Autodesk Inventor part; units mm, degrees
ref_plane "YZ Plane" through (0, 0, 0) normal (1, 0, 0) x (0, 1, 0)
ref_plane "XZ Plane" through (0, 0, 0) normal (0, 1, 0) x (-1, 0, 0)
ref_plane "XY Plane" through (0, 0, 0) normal (0, 0, 1) x (1, 0, 0)
sketch "Boceto1" plane through (0, 0, 0) normal (0, 0, 1) x (1, 0, 0)
  circle A0 centre (0, 0) radius 2.1
  line L0 (-12, 0) -> (12, 0)
  line L1 (0, 12) -> (0, -12)
  line L2 (0, 3.9) -> (-2.845, 3.9)
  line L3 (-2.845, 3.9) -> (-5.5, 6.555)
  line L4 (-5.5, 6.555) -> (-5.5, 8.195)
  line L5 (-5.5, 8.195) -> (-3.125, 8.195)
  line L6 (-3.125, 8.545) -> (-4.58, 10)
  line L7 (-4.58, 10) -> (-10, 10)
  line L8 (-10, 10) -> (-10, 4.58)
  line L9 (-10, 4.58) -> (-8.545, 3.125)
  line L10 (-8.195, 3.125) -> (-8.195, 5.4887)
  line L11 (-8.195, 5.4887) -> (-6.555, 5.4887)
  line L12 (-6.555, 5.4887) -> (-3.9, 2.8337)
  line L13 (-3.9, 2.8337) -> (-3.9, 0)
  line L14 (0, 3.9) -> (2.845, 3.9)
  line L15 (2.845, 3.9) -> (5.5, 6.555)
  line L16 (5.5, 6.555) -> (5.5, 8.195)
  line L17 (5.5, 8.195) -> (3.125, 8.195)
  line L18 (3.125, 8.545) -> (4.58, 10)
  line L19 (4.58, 10) -> (10, 10)
  line L20 (10, 10) -> (10, 4.58)
  line L21 (10, 4.58) -> (8.545, 3.125)
  line L22 (8.2079, 3.125) -> (8.195, 5.4887)
  line L23 (8.195, 5.4887) -> (6.555, 5.4887)
  line L24 (6.555, 5.4887) -> (3.9, 2.8337)
  line L25 (3.9, 2.8337) -> (3.9, 0)
  line L26 (0, -3.9) -> (-2.845, -3.9)
  line L27 (-2.845, -3.9) -> (-5.5, -6.555)
  line L28 (-5.5, -6.555) -> (-5.5, -8.195)
  line L29 (-5.5, -8.195) -> (-3.125, -8.195)
  line L30 (-3.125, -8.545) -> (-4.58, -10)
  line L31 (-4.58, -10) -> (-10, -10)
  line L32 (-10, -10) -> (-10, -4.58)
  line L33 (-10, -4.58) -> (-8.545, -3.125)
  line L34 (-8.195, -3.125) -> (-8.195, -5.4887)
  line L35 (-8.195, -5.4887) -> (-6.555, -5.4887)
  line L36 (-6.555, -5.4887) -> (-3.9, -2.8337)
  line L37 (-3.9, -2.8337) -> (-3.9, 0)
  line L38 (10, -10) -> (10, -4.58)
  line L39 (4.58, -10) -> (10, -10)
  line L40 (3.125, -8.545) -> (4.58, -10)
  line L41 (5.5, -8.195) -> (3.125, -8.195)
  line L42 (5.5, -6.555) -> (5.5, -8.195)
  line L43 (2.845, -3.9) -> (5.5, -6.555)
  line L44 (0, -3.9) -> (2.845, -3.9)
  line L45 (3.9, -2.8337) -> (3.9, 0)
  line L46 (6.555, -5.4887) -> (3.9, -2.8337)
  line L47 (8.195, -5.4887) -> (6.555, -5.4887)
  line L48 (8.195, -3.125) -> (8.195, -5.4887)
  line L49 (10, -4.58) -> (8.545, -3.125)
  line L50 (-3.125, 8.195) -> (-3.125, 8.545)
  line L51 (-8.195, 3.125) -> (-8.545, 3.125)
  line L52 (3.125, 8.195) -> (3.125, 8.545)
  line L53 (8.195, 3.125) -> (8.545, 3.125)
  line L54 (-3.125, -8.195) -> (-3.125, -8.545)
  line L55 (-8.195, -3.125) -> (-8.545, -3.125)
  line L56 (3.125, -8.195) -> (3.125, -8.545)
  line L57 (8.195, -3.125) -> (8.545, -3.125)
  dimension "d0" = 4.2
  dimension "d1" = 24
  dimension "d2" = 24
  dimension "d3" = 90
  dimension "d5" = 20
  dimension "d11" = 90
  dimension "d18" = 20
  dimension "d29" = 1.5
  dimension "d30" = 1.64
  dimension "d37" = 1.64
  dimension "d42" = 7.8
  dimension "d44" = 11
  dimension "d45" = 9.16
  dimension "d46" = 9.16
  dimension "d47" = 6.25
  dimension "d48" = 6.25
  dimension "d49" = 0.35
  dimension "d51" = 7.8
  dimension "d52" = 0.35
  dimension "d53" = 1.8
extrude "Extrusión1" add sketch "Boceto1" against normal blind 200 contours L0 L45 L46 L47 L48 L57 L49 L38 L39 L40 L56 L41 L42 L43 L44 L1 A0 | A0 L1 L14 L15 L16 L17 L52 L18 L19 L20 L21 L53 L22 L23 L24 L25 L0 | A0 L0 L13 L12 L11 L10 L51 L9 L8 L7 L6 L50 L5 L4 L3 L2 L1 | L1 L26 L27 L28 L29 L54 L30 L31 L32 L33 L55 L34 L35 L36 L37 L0 A0
fillet "Empalme1" radius 0.5 4 edges at (10, 10, -100) (-10, 10, -100) (10, -10, -100) (-10, -10, -100)
properties part number "Perfil2020" material "Aluminio 6061"
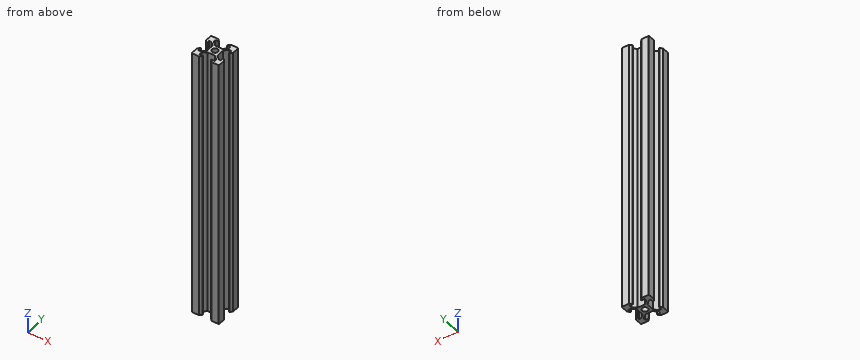
Could you check a few things on this model? Use its own coordinates, in mm. Round coordinates to 2 decimals unless told otherwise and drop trailing zeros. Loops run counter-clockwise (first coordinate to the right, second up) from the corner with the lowest first, then second, coordinate; pieces in that order, holes last. Notation, with made-up numbers: M 31.25,5.5 L 75.25,5.5 A18 ccw 75.25,14.5 Z; hole C 8,81.25 d2. An arc over 180 degrees is marked long. Put each result on its own line as item: value.
Q1. I need wall thicknesses on probe 1 along X at (y, z) = (0, -88); probe 2 along X at (y, z) = (5, -35.5) (3 decimals). Which ranges of each line are inside material? Lowest first, please.
Check result:
probe 1: -3.9 to -2.1, 2.1 to 3.9
probe 2: -10 to -8.195, -6.066 to -3.945, 3.945 to 6.066, 8.198 to 10
Q2. For pin 1 (6.5 mm diameter, centred on x = -1, z = -61, fed in from +Y); pin 2 (1.9 mm diameter, centred on y = -3.5, z = -141, fed in from +X); pin 3 (6 mm diameter, centred on y = -0.5, z = -76.5, fed in from +X), each with a flat end and sliding along its axis, tell me the tip position at first contact or that it passes through.
Check result:
pin 1: y = 9.67
pin 2: x = 9.87
pin 3: x = 8.92
Q3. Imagine slicing it at A-A (y = 0). Write out the boundary of the cut face in (x, z), then the cut area to 3 significant figures.
Check result:
outline: M -3.9,-200 L -2.1,-200 L -2.1,0 L -3.9,0 Z; M 2.1,-200 L 3.9,-200 L 3.9,0 L 2.1,0 Z
area: 720 mm2
